from build123d import *

# Parameters (mm, degrees)
SKETCH1_W           = 63.5
SKETCH1_H           = 88.9
BOSS_EXTRUDE1_DEPTH = 10.16
FILLET1_R           = 7.62
CUT_EXTRUDE1_DEPTH  = 8.128
SKETCH3_W           = 5.08
SKETCH3_H           = 5.08
SKETCH3_R           = 3.175
CUT_EXTRUDE2_DEPTH  = 12.7


with BuildPart() as part:
    # Sketch1 → Boss-Extrude1 (new body)
    with BuildSketch(Plane.XY):
        with Locations((31.75, -44.45)):
            Rectangle(SKETCH1_W, SKETCH1_H)
    extrude(amount=BOSS_EXTRUDE1_DEPTH)

    # Fillet1
    fillet1_edges = [part.edges().sort_by_distance(p)[0] for p in [
        (0, 0, 5.08),
        (63.5, 0, 5.08),
        (63.5, -88.9, 5.08),
        (0, -88.9, 5.08),
    ]]
    fillet(fillet1_edges, radius=FILLET1_R)

    # Sketch2 → Cut-Extrude1 (cut)
    with BuildSketch(Plane.XY.offset(10.16)):
        with BuildLine():
            Line((7.62, -2.54), (55.88, -2.54))
            ThreePointArc((55.88, -2.54), (59.472102448, -4.027897552), (60.96, -7.62))
            Line((60.96, -7.62), (60.96, -81.296436042))
            ThreePointArc((60.96, -81.296436042), (59.476916454, -84.876916454), (55.896436042, -86.36))
            Line((55.896436042, -86.36), (7.603563958, -86.36))
            ThreePointArc((7.603563958, -86.36), (4.023083546, -84.876916454), (2.54, -81.296436042))
            Line((2.54, -81.296436042), (2.54, -7.62))
            ThreePointArc((2.54, -7.62), (4.027897552, -4.027897552), (7.62, -2.54))
        make_face()
    extrude(amount=-CUT_EXTRUDE1_DEPTH, mode=Mode.SUBTRACT)

    # Sketch3 → Cut-Extrude2 (cut)
    with BuildSketch(Plane(origin=(0, 0, 0), x_dir=(-1, 0, 0), z_dir=(0, 0, -1))):
        with Locations((-33.528, -73.66)):
            Rectangle(SKETCH3_W, SKETCH3_H)
        with Locations((-11.43, -25.4)):
            Circle(SKETCH3_R)
    extrude(amount=-CUT_EXTRUDE2_DEPTH, mode=Mode.SUBTRACT)


solid = part.part
Design review of the part built by this model. Coordinates are the model's own, in mm. A direction names the side the tool comes from. Round coordinates to 2 decimals unless told otherwise and drop trailing zeros. Write each loop counter-clockwise with the first axis right and the second up, starting at its lowest first coordinate (ties: lowest second). Pieces come first, ordered by that corner, then holes. Notation, with made-up numbers: (20, 28.25) - (48, 28.25) arc R28 cw to (48, 61.25) - close; hole circle Ø5 at (-18.75, -30.5). An arc over 180 degrees is marked (long way). Return JSON: item names as keys, results as strings. Group by question number.
Item 1: We need section D-D on y = -40. Write out the cut boundary in (x, z), and give its area (3 significant figures).
Item 2: For probe 1 along Y at (x, z) = (11.43, 0.75) (3 decimals); probe 2 along Y at (x, z) = (55.5, 9); probe 3 along X at (y, z) = (-74, 9), list the stretches that pass through material, from the lowest coordinate up. Write a range as [from, to].
Item 3: The part is to be moulded in two halves that separate along X. For faces 4 (the face through (61.327, -2.291, 5.151)), 5 (the face through (60.96, -44, 6)), 6 (the face through (2.173, -2.291, 5.151)), 7 (the face through (11.84, -22.25, 1)), say which applies: pulls with the +X half, pulls with the -X half, needs draft (parallel to the pull), parting line crosses it, or undercut.
Item 4: We need section B-B on x = 11.43. Write out the cut boundary in (y, z) (3 decimals).
Item 5: Insertion check: P1, Ø8, axis at x = 22, y = -38, coming from the +Z side. The pin has a flat end and moves straight along its axis. Give the tip position at first contact, or say it passes through.
Item 6: We need section C-C on z = 3. Write out the cut boundary in (x, y), and give its area (3 significant figures).
Item 7: We need section A-A on y = -73. Write out the cut boundary in (x, z).
Item 8: Machinability: for faces 1 (the face through (63.5, -45, 5)), 2 (the face through (4.063, -84.916, 6.153)), 3 (the face through (36.068, -74, 1)), which of the approach directions +Z, -Z, +X, -X, +Y, -Y give a long, thin tool a straight path to every point of the face, cutting with its end or side? Answer none if there is none.
Model answer:
{
 "1": {"outline": "(0, 0) - (63.5, 0) - (63.5, 10.16) - (60.96, 10.16) - (60.96, 2.03) - (2.54, 2.03) - (2.54, 10.16) - (0, 10.16) - close", "area": "170 mm²"},
 "2": {"probe 1": "y = [-88.9, -28.575], [-22.225, 0]", "probe 2": "y = [-88.9, -86.36], [-2.54, 0]", "probe 3": "x = [0, 2.54], [60.96, 63.5]"},
 "3": {"face 4": "pulls with the +X half", "face 5": "undercut", "face 6": "pulls with the -X half", "face 7": "undercut"},
 "4": {"outline": "(-88.9, 0) - (-28.575, 0) - (-28.575, 2.032) - (-86.36, 2.032) - (-86.36, 10.16) - (-88.9, 10.16) - close; (-22.225, 0) - (0, 0) - (0, 10.16) - (-2.54, 10.16) - (-2.54, 2.032) - (-22.225, 2.032) - close"},
 "5": {"P1": "stops at z = 2.03"},
 "6": {"outline": "(0, -81.28) arc R7.62 ccw to (7.62, -88.9) - (55.88, -88.9) arc R7.62 ccw to (63.5, -81.28) - (63.5, -7.62) arc R7.62 ccw to (55.88, 0) - (7.62, 0) arc R7.62 ccw to (0, -7.62) - close; hole (2.54, -81.3) arc R5.06 ccw to (7.6, -86.36) - (55.9, -86.36) arc R5.06 ccw to (60.96, -81.3) - (60.96, -7.62) arc R5.08 ccw to (55.88, -2.54) - (7.62, -2.54) arc R5.08 ccw to (2.54, -7.62) - close", "area": "721 mm²"},
 "7": {"outline": "(0, 0) - (30.99, 0) - (30.99, 2.03) - (2.54, 2.03) - (2.54, 10.16) - (0, 10.16) - close; (36.07, 0) - (63.5, 0) - (63.5, 10.16) - (60.96, 10.16) - (60.96, 2.03) - (36.07, 2.03) - close"},
 "8": {"face 1": "+Z, -Z, +X, +Y, -Y", "face 2": "+Z", "face 3": "+Z, -Z"}
}
